Geometry check sheet. Reference: drawing and pictorial views, mm from the part's lowest x, y, z. Round coordinates to 2 decimals unless told otherwise and drop trailing zeros. Write each loop counter-clockwise with the first axis right and the second up, starting at its lowest first coordinate (ties: lowest second). Pieces come first, ordered by that corner, then holes. Notation, with made-up numbers: M 53.25,1 L 89.25,1 A22 cw 89.25,21 Z; hole C 33,28 d4. An arc over 180 degrees is marked long. Answer in a Markdown table with one row per item. Add a question column.
1. Material ranges on probe 1 along Y at (x, z) = (19, 2.15); probe 2 along Y at (x, z) = (68, 1.3); probe 3 along X at (y, z) = (8.5, 0.8), recorded low to high.
2. Sectioned sample at A-A on x = 56. Record the cut outline in (y, z).
3. Sectioned sample at C-C on z = 0.8. Count the separate pieces of the cut face and the enclosed holes in it, plus the area to 3 significant figures.
4. Sectioned sample at B-B on y = 55.5. Record the cut outline in (x, z).
5. Go/stop test with flat-tipped pins: pin 1 Ø3.5 at (x, y) = (56, 55.5) entering from +Z; pin 2 Ø0.6 at (x, z) = (41, 1) entering from +Y. Record where each tip stops, or that it passes through.
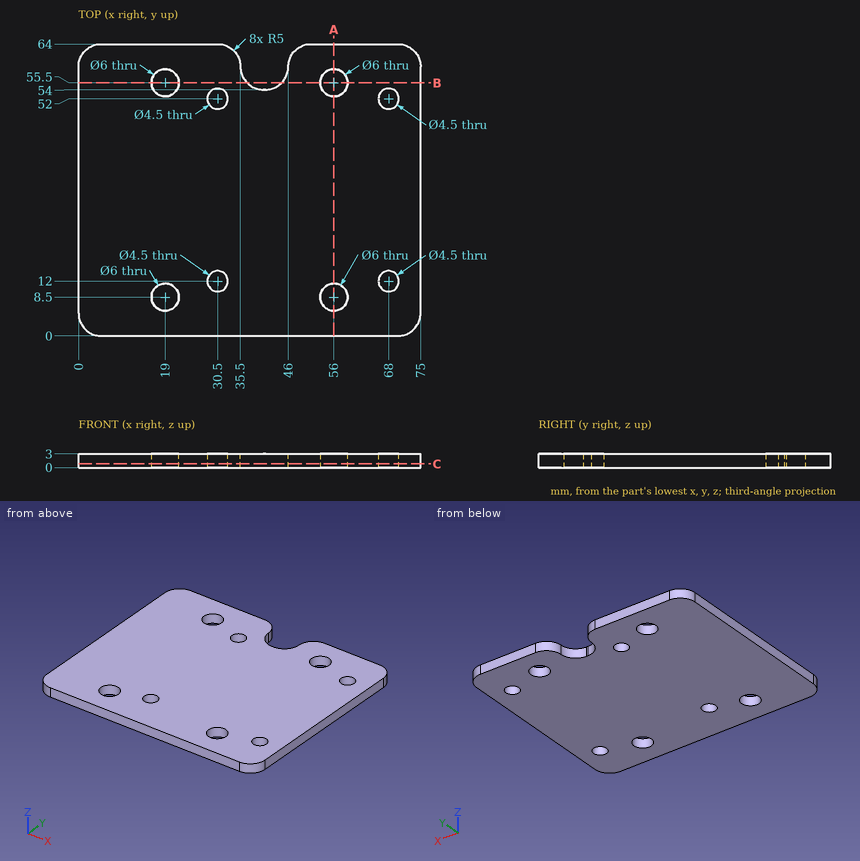
Geometry check:
| question | item | result |
|---|---|---|
| 1 | probe 1 | y = 0 to 5.5, 11.5 to 52.5, 58.5 to 64 |
| 1 | probe 2 | y = 0 to 9.75, 14.25 to 49.75, 54.25 to 64 |
| 1 | probe 3 | x = 0 to 16, 22 to 53, 59 to 75 |
| 2 | outline | M 0,0 L 5.5,0 L 5.5,3 L 0,3 Z; M 11.5,0 L 52.5,0 L 52.5,3 L 11.5,3 Z; M 58.5,0 L 64,0 L 64,3 L 58.5,3 Z |
| 3 | separate pieces | 1 |
| 3 | enclosed holes | 8 |
| 3 | area | 4,500 mm2 |
| 4 | outline | M 0,0 L 16,0 L 16,3 L 0,3 Z; M 22,0 L 36.93,0 L 36.93,3 L 22,3 Z; M 44.57,0 L 53,0 L 53,3 L 44.57,3 Z; M 59,0 L 75,0 L 75,3 L 59,3 Z |
| 5 | pin 1 | passes through |
| 5 | pin 2 | stops at y = 54.01 |
